Autodesk Inventor part; units mm, degrees
ref_plane "YZ Plane" through (0, 0, 0) normal (1, 0, 0) x (0, 1, 0)
ref_plane "XZ Plane" through (0, 0, 0) normal (0, 1, 0) x (-1, 0, 0)
ref_plane "XY Plane" through (0, 0, 0) normal (0, 0, 1) x (1, 0, 0)
sketch "Boceto1" plane through (0, 0, 0) normal (0, 0, 1) x (1, 0, 0)
  line L0 (29.9998, -9.9999) -> (-15.0002, -9.9999)
  line L1 (-15.0002, -9.9999) -> (-15.0002, 30.0001)
  line L2 (-15.0002, 30.0001) -> (29.9998, 30.0001)
  line L3 (29.9998, 30.0001) -> (29.9998, -9.9999)
  line L4 (-9.8002, -9.9999) -> (-4.883, -9.9999)
  line L5 (29.9998, 24.8001) -> (29.9998, 30.0001)
  line L6 (-4.8002, 30.0001) -> (-10.0002, 30.0001)
  point P0 (0, 0)
  dimension "d0" = 45
extrude "Extrusión1" add sketch "Boceto1" along normal blind 6
sketch "Boceto8" plane through (0, 0, 6) normal (0, 0, 1) x (1, 0, 0)
  circle A0 centre (19.9998, 0.0001) radius 2.5
  circle A1 centre (19.9998, 20.0001) radius 2.5
  circle A2 centre (-0.0002, 0.0001) radius 2.5
  circle A3 centre (-0.0002, 20.0001) radius 2.5
  circle A4 centre (19.9998, 20.0001) radius 2.75
  circle A5 centre (-0.0002, 20.0001) radius 2.75
  circle A6 centre (-0.0002, 0.0001) radius 2.75
  circle A7 centre (19.9998, 0.0001) radius 2.75
  point P0 (0, 0)
  dimension "d28" = 5.5
  dimension "d29" = 5.5
  dimension "d30" = 5.5
  dimension "d31" = 5.5
extrude "Extrusión8" cut sketch "Boceto8" against normal through all contours A0 | A1 | A2 | A3 | A4 | A5 | A6 | A7
sketch "Boceto9" plane through (0, 0, 6) normal (0, 0, 1) x (1, 0, 0)
  circle A0 centre (19.9998, 0.0001) radius 2.75
  circle A1 centre (-0.0002, 0.0001) radius 2.75
  circle A2 centre (-0.0002, 20.0001) radius 2.75
  circle A3 centre (19.9998, 20.0001) radius 2.75
  circle A4 centre (19.9998, 0.0001) radius 5.75
  circle A5 centre (-0.0002, 0.0001) radius 2.75
  circle A6 centre (-0.0002, 0.0001) radius 5.75
  circle A7 centre (19.9998, 20.0001) radius 2.75
  circle A8 centre (19.9998, 20.0001) radius 5.75
  circle A9 centre (-0.0002, 20.0001) radius 5.75
  point P0 (0, 0)
  dimension "d34" = 11.5
  dimension "d35" = 11.5
  dimension "d36" = 11.5
  dimension "d37" = 11.5
extrude "Extrusión9" cut sketch "Boceto9" against normal blind 3
properties part number "MONTURA LCD"
Verification items for the finished model (mm, model axes). A direction names the side the tool comes from. Round coordinates to 2 decimals unless told otherwise and drop trailing zeros. Order: outer loops, then holes, each group sorted by start corner. A loop starts at its lowest first (then second) coordinate and runs counter-clockwise, first axis right, second up. Notation, with made-up numbers: (-37.75, -10) - (-22.75, -10) arc R17 cw to (-22.75, 9) - close; hole circle Ø5 at (-5.75, 84.5). An arc over 180 degrees is marked (long way). Use CSV: the item, a comma, the result in double quotes. Start each with the question number.
1) Section check B-B, the plane y = -1. Record the cut outline in (x, z).
2) Section check D-D, the plane y = 23.5. Record the cut outline in (x, z), plus the area to 3 significant figures.
3) Mould release check, pull along X, two halves, no side actions. Record for faces 1 (the flat face through (30, 10, 3)), 2 (the cylindrical face through (25.311, -2.202, 4.521)), 3 (the cylindrical face through (-0.75, 25.7, 4.52)), 4 (the flat face through (7, 30, 3)): +X half, -X half, draft (parallel to the pull), parting line (faces both ways), or undercut.
4) Section check A-A, the plane x = 0. Record the cut outline in (y, z).
5) Go/stop test with flat-tipped pins: P1, Ø3.5, axis at x = 22.5, y = 20.5, coming from the +Z side; P2, Ø3.5, axis at x = 20, y = 0, coming from the -Z side. Record where each tip stops, or that it passes through.
6) Thickness scan on L1, parallel to X at y = 0, z = 2.3; L2, parallel to Y at x = 3.5, z = 4.65; L3, parallel to Y at x = 24.5, z = 4.9. Record the ranges inside material, lowest first.
7) Section check C-C, the plane z = 5.4. Record the cut outline in (x, y), plus the area to 3 significant figures.
8) Access from +Z, -Z, +X, -X, +Y, -Y to the whole of each face (thin tool, end or side, straight path). Record for faces 5 (the cylindrical face through (5.484, 1.727, 4.521)), 6 (the cylindrical face through (-0.358, 22.727, 1.521)).
Answers:
1,outline,"(-15, 0) - (-2.56, 0) - (-2.56, 3) - (-5.66, 3) - (-5.66, 6) - (-15, 6) - close; (2.56, 0) - (17.44, 0) - (17.44, 3) - (14.34, 3) - (14.34, 6) - (5.66, 6) - (5.66, 3) - (2.56, 3) - close; (22.56, 0) - (30, 0) - (30, 6) - (25.66, 6) - (25.66, 3) - (22.56, 3) - close"
2,outline,"(-15, 0) - (30, 0) - (30, 6) - (24.56, 6) - (24.56, 3) - (15.44, 3) - (15.44, 6) - (4.56, 6) - (4.56, 3) - (-4.56, 3) - (-4.56, 6) - (-15, 6) - close"
2,area,"215 mm²"
3,face 1,"+X half"
3,face 2,"undercut"
3,face 3,"undercut"
3,face 4,"draft"
4,outline,"(-10, 0) - (-2.75, 0) - (-2.75, 3) - (-5.75, 3) - (-5.75, 6) - (-10, 6) - close; (2.75, 0) - (17.25, 0) - (17.25, 3) - (14.25, 3) - (14.25, 6) - (5.75, 6) - (5.75, 3) - (2.75, 3) - close; (22.75, 0) - (30, 0) - (30, 6) - (25.75, 6) - (25.75, 3) - (22.75, 3) - close"
5,P1,"stops at z = 3"
5,P2,"passes through"
6,L1,"x = -15 to -2.75, 2.75 to 17.25, 22.75 to 30"
6,L2,"y = -10 to -4.56, 4.56 to 15.44, 24.56 to 30"
6,L3,"y = -10 to -3.58, 3.58 to 16.42, 23.58 to 30"
7,outline,"(-15, -10) - (30, -10) - (30, 30) - (-15, 30) - close; hole circle Ø11.5 at (0, 0); hole circle Ø11.5 at (0, 20); hole circle Ø11.5 at (20, 0); hole circle Ø11.5 at (20, 20)"
7,area,"1,380 mm²"
8,face 5,"+Z"
8,face 6,"+Z, -Z"
